Input: part model. Units: mm. Frame: model coordinates. A direction names the side the tool comes from. Round coordinates to 2 decimals unless told otherwise and drop trailing zeros. Loops run counter-clockwise (first coordinate to the right, second up) from the corner with the lowest first, then second, coordinate; pieces in that order, holes last.
1) Section A-A, the plane x = 32.5. Return loops of the section in (y, z).
2) Section B-B, the plane y = 25. Return loops of the section in (x, z) (3 decimals), and give its area (3 significant figures).
3) Ray query, line 1 along Y through (x, z) = (-7.75, 1.15); line 2 along Z through (x, y) = (32.5, 2.25); line 3 along Y through (x, z) = (15.5, 2). Return the intervals inside material, ascending.
4) Draft query along X for faces 1 (the face through (7, 0, 4)), 2 (the face through (-4.01, 6.94, 6.03)), 3 (the face through (28.575, 27, 4)). Return one class per face: pulls with the +X half, pulls with the -X half, needs draft (parallel to the pull), parting line crosses it, or undercut.
5) Access query for faces 4 (the face through (0, 21, 4)), 5 (the face through (7, 3, 23)), 6 (the face through (7, 43, 8)). Directions: +Z, -Z, +X, -X, +Y, -Y. A direction counts if a zero-diameter tool reaches every point of the face in a straight line with its end or side. Return the directions, or none.
6) Section C-C, the plane x = 15.5. Return loops of the section in (y, z).
7) First-contact query: pin 1 (4 mm diameter, centred on x = 7.75, y = 11.58, fed in from +Z); pin 2 (2 mm diameter, centred on y = 40, z = 5.5, fed in from +X) (3 decimals); pin 3 (6 mm diameter, centred on x = 30.5, y = 37.5, fed in from +Z). Flat tips, straight axial feed; report the tip coordinate or a pass-through.
8) Section D-D, the plane z = 2.5. Return loops of the section in (x, y) (3 decimals).
from build123d import *

# Parameters (mm, degrees)
SKETCH3_W                                       = 57.15
SKETCH3_H                                       = 50
BOSS_EXTRUDE1_DEPTH                             = 8
SKETCH3_3_R                                     = 1.5
SKETCH3_3_R_2                                   = 8
CUT_EXTRUDE2_DEPTH                              = 10
SKETCH4_R                                       = 18.5
CUT_EXTRUDE3_DEPTH                              = 4
BOSS_EXTRUDE2_DEPTH                             = 15
BOSS_EXTRUDE2_DEPTH_BACK                        = 23
SKETCH6_W                                       = 80
SKETCH6_H                                       = 5
CSK_FOR_M3_FLAT_HEAD_MACHINE_SCREW1_D           = 3.4
CSK_FOR_M3_FLAT_HEAD_MACHINE_SCREW1_CSINK_D     = 6.3
CSK_FOR_M3_FLAT_HEAD_MACHINE_SCREW1_CSINK_ANGLE = 90
CUT_EXTRUDE8_REACH                              = 66.452
SKETCH14_W                                      = 15.24
SKETCH14_H                                      = 38
CUT_EXTRUDE8_DIRECTION_2_DEPTH                  = 45


with BuildPart() as part:
    # Sketch3 → Boss-Extrude1 (new body)
    with BuildSketch(Plane.XY):
        with Locations((0, 25)):
            Rectangle(SKETCH3_W, SKETCH3_H)
    extrude(amount=BOSS_EXTRUDE1_DEPTH)

    # Sketch3<3> → Cut-Extrude2 (cut)
    with BuildSketch(Plane.XY):
        with Locations(Location((-7.75, 38.423393759, 0), (0, 0, 180))):
            Circle(SKETCH3_3_R)
        with Locations(Location((7.75, 38.423393759, 0), (0, 0, 180))):
            Circle(SKETCH3_3_R)
        with Locations(Location((-7.75, 11.576606241, 0), (0, 0, 180))):
            Circle(SKETCH3_3_R)
        with Locations(Location((7.75, 11.576606241, 0), (0, 0, 180))):
            Circle(SKETCH3_3_R)
        with Locations(Location((15.5, 25, 0), (0, 0, 180))):
            Circle(SKETCH3_3_R)
        with Locations(Location((6.062177825, 28.499999999, 0), (0, 0, 180))):
            Circle(SKETCH3_3_R_2)
    extrude(amount=CUT_EXTRUDE2_DEPTH, mode=Mode.SUBTRACT)

    # Sketch4 → Cut-Extrude3 (cut)
    with BuildSketch(Plane.XY.offset(8)):
        with Locations((0, 25)):
            Circle(SKETCH4_R)
    extrude(amount=-CUT_EXTRUDE3_DEPTH, mode=Mode.SUBTRACT)

    # Sketch6 → Boss-Extrude2 (add, two sides: drawn at the far end of the back side and taken through both)
    with BuildSketch(Plane.XY.offset(8).offset(-BOSS_EXTRUDE2_DEPTH_BACK)):
        with Locations((0, 2.5)):
            Rectangle(SKETCH6_W, SKETCH6_H)
    extrude(amount=BOSS_EXTRUDE2_DEPTH + BOSS_EXTRUDE2_DEPTH_BACK)

    # CSK for M3 Flat Head Machine Screw1 (through all)
    with Locations(Plane(origin=(0, 5, 0), x_dir=(1, 0, 0), z_dir=(0, 1, 0))):
        with Locations((-32.5, 7.5), (-32.5, -15.5), (32.5, -15.5), (32.5, 7.5)):
            CounterSinkHole(CSK_FOR_M3_FLAT_HEAD_MACHINE_SCREW1_D / 2, CSK_FOR_M3_FLAT_HEAD_MACHINE_SCREW1_CSINK_D / 2, counter_sink_angle=CSK_FOR_M3_FLAT_HEAD_MACHINE_SCREW1_CSINK_ANGLE)

    # Sketch14 → Cut-Extrude8 (cut, up to next)
    with BuildSketch(Plane(origin=(0, 5, 0), x_dir=(1, 0, 0), z_dir=(0, 1, 0)), mode=Mode.PRIVATE) as cut_extrude8_sk1:
        with Locations((-32.38, -4)):
            Rectangle(SKETCH14_W, SKETCH14_H)
    cut_extrude8_tool1 = extrude(cut_extrude8_sk1.sketch, amount=-CUT_EXTRUDE8_REACH, mode=Mode.PRIVATE) & part.part
    add(cut_extrude8_tool1.solids().sort_by_distance((-32.38, 5, 4))[0], mode=Mode.SUBTRACT)

    # Sketch14 → Cut-Extrude8 direction 2 (cut)
    with BuildSketch(Plane(origin=(0, 5, 0), x_dir=(1, 0, 0), z_dir=(0, 1, 0))):
        with Locations((-32.38, -4)):
            Rectangle(SKETCH14_W, SKETCH14_H)
    extrude(amount=CUT_EXTRUDE8_DIRECTION_2_DEPTH, mode=Mode.SUBTRACT)


solid = part.part
Final values:
1. outline: (0, -15) - (5, -15) - (5, -10.65) - (3.55, -9.2) - (0, -9.2) - close; (0, -5.8) - (3.55, -5.8) - (5, -4.35) - (5, 12.35) - (3.55, 13.8) - (0, 13.8) - close; (0, 17.2) - (3.55, 17.2) - (5, 18.65) - (5, 23) - (0, 23) - close
2. outline: (-24.76, 0) - (-1.132, 0) - (-1.132, 4) - (-18.5, 4) - (-18.5, 8) - (-24.76, 8) - close; (13.256, 0) - (14, 0) - (14, 4) - (13.256, 4) - close; (17, 0) - (28.575, 0) - (28.575, 8) - (18.5, 8) - (18.5, 4) - (17, 4) - close
2. area: 209 mm2
3. line 1: y = 0 to 10.08, 13.08 to 36.92, 39.92 to 50
3. line 2: z = -15 to -9.2, -5.8 to 13.8, 17.2 to 23
3. line 3: y = 0 to 23.5, 26.5 to 50
4. face 1: needs draft
4. face 2: undercut
4. face 3: pulls with the +X half
5. face 4: +Z
5. face 5: +Z, +X, -X, +Y, -Y
5. face 6: +Z, +X, -X, +Y
6. outline: (0, -15) - (5, -15) - (5, 0) - (23.5, 0) - (23.5, 4) - (14.9, 4) - (14.9, 8) - (5, 8) - (5, 23) - (0, 23) - close; (26.5, 0) - (50, 0) - (50, 8) - (35.1, 8) - (35.1, 4) - (26.5, 4) - close
7. pin 1: stops at z = 4
7. pin 2: stops at x = 28.575
7. pin 3: stops at z = 8
8. outline: (-24.76, 0) - (40, 0) - (40, 5) - (28.575, 5) - (28.575, 50) - (-24.76, 50) - close; hole circle Ø3 at (-7.75, 11.577); hole circle Ø3 at (-7.75, 38.423); hole circle Ø16 at (6.062, 28.5); hole circle Ø3 at (7.75, 11.577); hole circle Ø3 at (7.75, 38.423); hole circle Ø3 at (15.5, 25)
